Autodesk Inventor part; units mm, degrees
ref_plane "YZ Plane" through (0, 0, 0) normal (1, 0, 0) x (0, 1, 0)
ref_plane "XZ Plane" through (0, 0, 0) normal (0, 1, 0) x (-1, 0, 0)
ref_plane "XY Plane" through (0, 0, 0) normal (0, 0, 1) x (1, 0, 0)
sketch "Sketch1" plane through (0, 0, 0) normal (1, 0, 0) x (0, 1, 0)
  line L0 (-12.7, 50.8) -> (12.7, 50.8)
  line L1 (25.4, 38.1) -> (25.4, -38.1)
  line L2 (12.7, -50.8) -> (-12.7, -50.8)
  line L3 (-25.4, -38.1) -> (-25.4, 38.1)
  line L4 (-25.4, 50.8) -> (25.4, -50.8) construction
  line L5 (25.4, 50.8) -> (-25.4, -50.8) construction
  arc A0 (25.4, 38.1) -> (12.7, 50.8) centre (12.7, 38.1) ccw
  arc A1 (-12.7, 50.8) -> (-25.4, 38.1) centre (-12.7, 38.1) ccw
  arc A2 (-25.4, -38.1) -> (-12.7, -50.8) centre (-12.7, -38.1) ccw
  arc A3 (12.7, -50.8) -> (25.4, -38.1) centre (12.7, -38.1) ccw
  point P0 (0, 0)
  dimension "d0" = 101.6
  dimension "d1" = 50.8
  dimension "d2" = 12.7
extrude "Extrusion1" add sketch "Sketch1" against normal blind 304.8
properties part number "Wood-3"
The listing builds one solid part. Answer for the finished solid, in the listing's coordinates (mm). Give positions to 0.01 mm unless a question says otherwise; leave off trailing zeros. Order: outer loops, then holes, each group sorted by start corner. A loop starts at its lowest first (then second) coordinate and runs counter-clockwise, first axis right, second up. Notation, with made-up numbers: (38, 0.25) - (97, 0.25) arc R21 ccw to (97, 10.25) - close; hole circle Ø8 at (21.25, 0.5). An arc over 180 degrees is marked (long way). Use one line per item in the form item = value. Start each with the question number.
(1) A flat-ended cylindrical pin translates along its axis: pin 1 Ø4 at (y, z) = (8, -29.5) entering from +X. Find the tip coordinate at first contact, or state that the pin passes through.
(2) A cutting plane is placed at B-B, the plane y = 20. Write down the section's boundary in (x, z), then the cut area to 3 significant figures.
(3) Consider line 1 (Y direction, x = -20.5, z = -39); line 2 (Z direction, x = -90.5, y = -23); line 3 (Z direction, x = -165.5, y = 17.5). Determine where each line is inside the solid, lowest interval first. Write a range as from..to.
(4) A cutting plane is placed at A-A, the plane x = -135.5. Write down the section's boundary in (y, z).
Ans:
q1.pin_1 = 0
q2.outline = (-304.8, -48.49) - (0, -48.49) - (0, 48.49) - (-304.8, 48.49) - close
q2.area = 29,600 mm^2
q3.line_1 = -25.37..25.37
q3.line_2 = -45.53..45.53
q3.line_3 = -49.86..49.86
q4.outline = (-25.4, -38.1) arc R12.7 ccw to (-12.7, -50.8) - (12.7, -50.8) arc R12.7 ccw to (25.4, -38.1) - (25.4, 38.1) arc R12.7 ccw to (12.7, 50.8) - (-12.7, 50.8) arc R12.7 ccw to (-25.4, 38.1) - close
